Input: part model. Units: mm. Frame: model coordinates. Face numbers are marked on the shaded views. A direction names the side the tool comes from. Coordinates: 2 decimals unless noted, no trailing zeros. Loops run counter-clockwise (first coordinate to the right, second up) from the corner with the lowest first, then second, coordinate; pieces in that order, holes last. Notation, with made-up numbers: (-8.5, -25.75) -> (30.5, -25.75) arc R16 cw to (30.5, -11.75) -> close; hole circle Ø4 at (15, -14). An arc over 180 degrees is marked (long way). Answer as a JSON object with one key per item and string values.
Autodesk Inventor part; units mm, degrees
ref_plane "YZ Plane" through (0, 0, 0) normal (1, 0, 0) x (0, 1, 0)
ref_plane "XZ Plane" through (0, 0, 0) normal (0, 1, 0) x (-1, 0, 0)
ref_plane "XY Plane" through (0, 0, 0) normal (0, 0, 1) x (1, 0, 0)
sketch "Sketch1" plane through (0, 0, 0) normal (0, 0, 1) x (1, 0, 0)
  circle A0 centre (0, 0) radius 2.159
  dimension "d0" = 4.318
extrude "Extrusion1" add sketch "Sketch1" along normal blind 10.16
sketch "Sketch2" plane through (0, 0, 0) normal (0, 0, -1) x (-1, 0, 0)
  circle A0 centre (0, 0) radius 2.159
  circle A1 centre (0, 0) radius 1.4986
  dimension "d3" = 2.9972
extrude "Extrusion2" add sketch "Sketch2" along normal blind 6.096 contours A1
sketch "Sketch3" plane through (0, 0, 0) normal (0, 0, -1) x (-1, 0, 0)
  circle A0 centre (0, 0) radius 2.159
  circle A1 centre (0, 0) radius 5.461
  dimension "d6" = 10.922
extrude "Extrusion3" add sketch "Sketch3" against normal blind 5
sketch "Sketch4" plane through (0, 0, 5) normal (0, 0, 1) x (1, 0, 0)
  circle A0 centre (0, 0) radius 2.159
  line L0 (-7.6454, 0) -> (7.6454, 0)
  point P0 (3.81, 0)
  point P1 (-1.905, 3.2996)
  point P2 (-1.905, -3.2996)
  dimension "d9" = 3.81
  dimension "d12" = 360
hole "Hole1" at (-1.905, 3.2996, 5) at (-1.905, -3.2996, 5) direction (0, 0, -1) diameter 1.524 end through all
properties part number "Post"
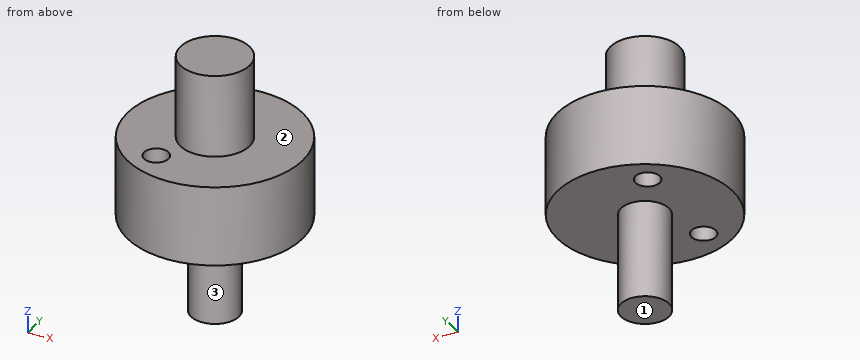
1. Section query A-A (y = 2.75). Return loops of the section in (x, z), plus the area to 3 significant figures.
Reply:
{"outline": "(-4.72, 0) -> (-2.43, 0) -> (-2.43, 5) -> (-4.72, 5) -> close; (-1.38, 0) -> (4.72, 0) -> (4.72, 5) -> (-1.38, 5) -> close", "area": "41.9 mm2"}
2. Pin query (flat end, axial travel): P1, Ø1, axis at y = -2.5, z = -2, coming from the +X side; P2, Ø1.5, axis at x = -1, z = 3.5, coming from the +Y side; P3, Ø3.5, axis at x = -1.5, y = 2, coming from the -Z side; P4, Ø4, axis at x = 2.5, z = 2, coming from the -Y side. Return the tip coordinate at first contact, or that it passes through.
Reply:
{"P1": "passes through", "P2": "stops at y = 5.46", "P3": "stops at z = -6.1", "P4": "stops at y = -5.44"}
3. Section query B-B (x = 0). Return loops of the section in (y, z).
Reply:
{"outline": "(-5.46, 0) -> (-1.5, 0) -> (-1.5, -6.1) -> (1.5, -6.1) -> (1.5, 0) -> (5.46, 0) -> (5.46, 5) -> (2.16, 5) -> (2.16, 10.16) -> (-2.16, 10.16) -> (-2.16, 5) -> (-5.46, 5) -> close"}
4. Section query D-D (z = 0.5). Return loops of the section in (x, y) (3 decimals), plus the area to 3 significant figures.
Reply:
{"outline": "circle Ø10.922 at (0, 0); hole circle Ø1.524 at (-1.905, -3.3); hole circle Ø1.524 at (-1.905, 3.3)", "area": "90.0 mm2"}
5. Access query for the marked faces 1, 2 and 3. Directions: +Z, -Z, +X, -X, +Y, -Y. A direction counts if a zero-diameter tool reaches every point of the face in a straight line with its end or side. Return the directions, or none.
Reply:
{"face 1": "-Z, +X, -X, +Y, -Y", "face 2": "+Z", "face 3": "-Z"}
6. Line query: line 1 along Y through (x, z) = (-2.5, 3.25); line 2 along Z through (x, y) = (-1.5, 4.5); line 3 along X through (y, z) = (-3.5, 2.5). Output: solid intervals per line, ascending.
Reply:
{"line 1": "y = -4.86 to -3.78, -2.82 to 2.82, 3.78 to 4.86", "line 2": "z = 0 to 5", "line 3": "x = -4.19 to -2.64, -1.17 to 4.19"}
